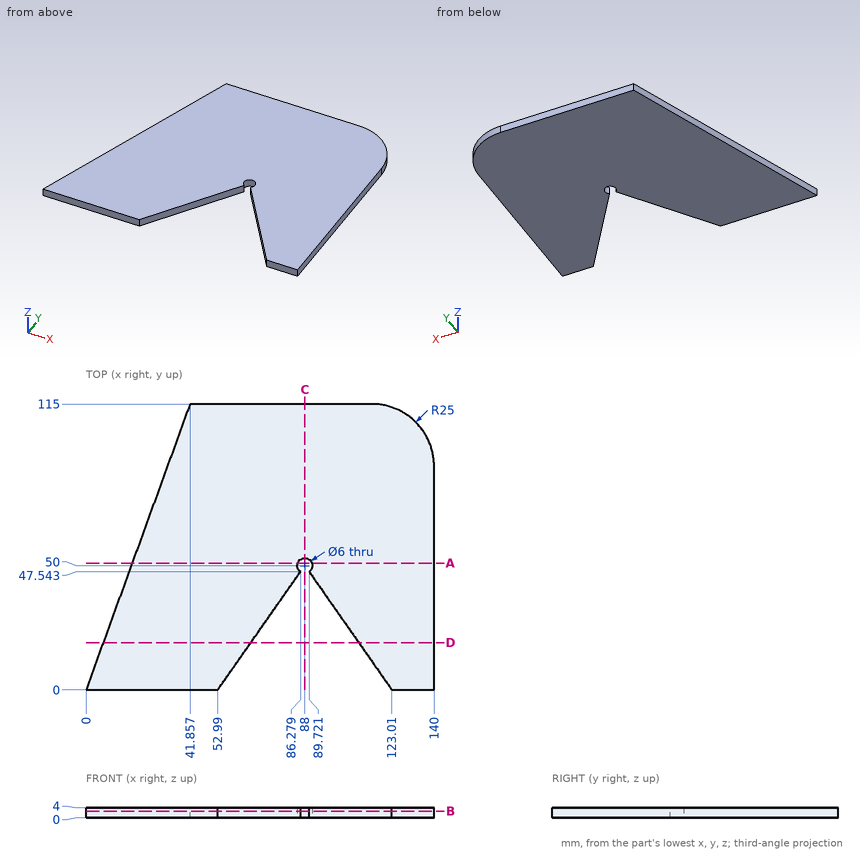
Here's the drawing with two shaded views (mm, measured from the low corner). I have some questions. Coordinates: 2 decimals unless noted, no trailing zeros. Order: outer loops, then holes, each group sorted by start corner. A loop starts at its lowest first (then second) coordinate and runs counter-clockwise, first axis right, second up. Notation, with made-up numbers: (14.25, -1) - (45.25, -1) arc R6 ccw to (45.25, 4) - close; hole circle Ø1 at (-35, 22.5). An arc over 180 degrees is marked (long way). Use CSV: the item, a comma, the result in double quotes. Start each with the question number.
1. Suppose I cut it at C-C on x = 88. List the corners of the cut face in (y, z) for me, then the cut area to 3 significant figures.
2. Suppose I cut it at A-A on y = 51. List the corners of the cut face in (x, z) for me, then the cut area to 3 significant figures.
3. Suppose I cut it at B-B on z = 2.7. List the corners of the cut face in (x, y) for me.
4. Please list where these lines run through material, in increasing order: line 1 (Y direction, x = 88, z = 2); line 2 (X direction, y = 50, z = 2.9); line 3 (X direction, y = 41, z = 2.9). Write a range as from..to.
5. Suppose I cut it at D-D on y = 19. List the corners of the cut face in (x, z) for me (1 decimal).
6. I'm going to push a flat-ended pin straight in: pin 1 (7 mm diameter, centred on x = 88, y = 50, fed in from -Z). Where does the tip first touch, or does it pass through?
Output:
1,outline,"(53, 0) - (115, 0) - (115, 4) - (53, 4) - close"
1,area,"248 mm2"
2,outline,"(18.56, 0) - (85.17, 0) - (85.17, 4) - (18.56, 4) - close; (90.83, 0) - (140, 0) - (140, 4) - (90.83, 4) - close"
2,area,"463 mm2"
3,outline,"(0, 0) - (52.99, 0) - (86.28, 47.54) arc R3 cw (long way) to (89.72, 47.54) - (123.01, 0) - (140, 0) - (140, 90) arc R25 ccw to (115, 115) - (41.86, 115) - close"
4,line 1,"y = 53..115"
4,line 2,"x = 18.2..85, 91..140"
4,line 3,"x = 14.92..81.7, 94.3..140"
5,outline,"(6.9, 0) - (66.3, 0) - (66.3, 4) - (6.9, 4) - close; (109.7, 0) - (140, 0) - (140, 4) - (109.7, 4) - close"
6,pin 1,"stops at z = 0"
